Read the model definition and answer for the solid it produces. Units are mm, in the model's axes. A direction names the side the tool comes from. Give positions to 0.01 mm unless a question says otherwise; leave off trailing zeros. Order: outer loops, then holes, each group sorted by start corner. A loop starts at its lowest first (then second) coordinate and runs counter-clockwise, first axis right, second up.
```python
from build123d import *

# Parameters (mm, degrees)
F0_W      = 177.8
F0_H      = 138.684
F1_DEPTH  = 25.4
F2_W      = 177.8
F2_H      = 138.684
F2_W_2    = 161.3722443581
F2_H_2    = 112.8829941154
F3_DEPTH  = 19.05
F4_W      = 141.4277553558
F4_H      = 98.9994257689
F5_DEPTH  = 19.05
F6_R      = 25.4
F7_R      = 4.7625
F8_DEPTH  = 6.351
F9_SIZE   = 1.524
F10_R     = 1.5875
F11_DEPTH = 6.351
F12_SIZE  = 1.778


with BuildPart() as f1:
    # F0 (on Front) → F1 (new body)
    with BuildSketch(Plane.XZ):
        Rectangle(F0_W, F0_H)
    extrude(amount=F1_DEPTH)

    # F2 (on face) → F3 (cut)
    with BuildSketch(Plane(origin=(0, 0, 0), x_dir=(-1, 0, 0), z_dir=(0, 1, 0))):
        Rectangle(F2_W, F2_H)
        Rectangle(F2_W_2, F2_H_2, mode=Mode.SUBTRACT)
    extrude(amount=-F3_DEPTH, mode=Mode.SUBTRACT)

    # F4 (on face) → F5 (cut)
    with BuildSketch(Plane.XZ.offset(25.4)):
        Rectangle(F4_W, F4_H)
    extrude(amount=-F5_DEPTH, mode=Mode.SUBTRACT)

    # F6
    f6_edges = [f1.edges().sort_by_distance(p)[0] for p in [
        (88.9, -22.225, 69.342),
        (88.9, -22.225, -69.342),
        (-88.9, -22.225, -69.342),
        (-88.9, -22.225, 69.342),
        (-70.713878, -15.875, 49.499713),
        (70.713878, -15.875, 49.499713),
        (70.713878, -15.875, -49.499713),
        (-70.713878, -15.875, -49.499713),
        (80.686122, -9.525, -56.441497),
        (80.686122, -9.525, 56.441497),
        (-80.686122, -9.525, -56.441497),
        (-80.686122, -9.525, 56.441497),
    ]]
    fillet(f6_edges, radius=F6_R)

    # F7 (on face) → F8 (cut, through all)
    with BuildSketch(Plane.XZ.offset(6.35)):
        with Locations((-25.4, 23.863709036)):
            Circle(F7_R)
        with Locations((25.4, 23.863709036)):
            Circle(F7_R)
        with Locations((0, -19.9294611812)):
            Circle(F7_R)
    extrude(amount=-F8_DEPTH, mode=Mode.SUBTRACT)

    # F9
    f9_edges = [f1.edges().sort_by_distance(p)[0] for p in [
        (0, -25.4, -49.499713),
        (70.713878, -25.4, 0),
        (-88.9, -25.4, 0),
        (-81.460512, -25.4, -61.902512),
        (0, 0, -56.441497),
        (88.9, -25.4, 0),
        (81.460512, -25.4, 61.902512),
        (81.460512, -25.4, -61.902512),
        (0, -25.4, -69.342),
        (0, -25.4, 69.342),
        (-81.460512, -25.4, 61.902512),
        (-63.27439, -25.4, -42.060225),
        (63.27439, -25.4, -42.060225),
        (-70.713878, -25.4, 0),
        (-63.27439, -25.4, 42.060225),
        (63.27439, -25.4, 42.060225),
        (0, -25.4, 49.499713),
        (-80.686122, 0, 0),
        (-73.246634, 0, 49.002009),
        (-73.246634, 0, -49.002009),
        (0, 0, 56.441497),
        (73.246634, 0, 49.002009),
        (73.246634, 0, -49.002009),
        (80.686122, 0, 0),
    ]]
    chamfer(f9_edges, length=F9_SIZE)

    # F10 (on face) → F11 (cut, through all)
    with BuildSketch(Plane(origin=(0, -19.05, 0), x_dir=(-1, 0, 0), z_dir=(0, 1, 0))):
        with Locations((-79.0948867798, 54.6215597034)):
            Circle(F10_R)
        with Locations((79.6314403415, 54.6215597034)):
            Circle(F10_R)
        with Locations((79.6314403415, -54.8539970577)):
            Circle(F10_R)
        with Locations((-79.0948867798, -54.8539970577)):
            Circle(F10_R)
    extrude(amount=-F11_DEPTH, mode=Mode.SUBTRACT)

    # F12
    f12_edges = [f1.edges().sort_by_distance(p)[0] for p in [
        (-78.04394, -25.4, 54.62156),
        (80.682387, -25.4, 54.62156),
        (80.682387, -25.4, -54.853997),
        (-78.04394, -25.4, -54.853997),
    ]]
    chamfer(f12_edges, length=F12_SIZE)


solid = f1.part
```
1) Consider L1, parallel to X at y = -8.75, z = -5; L2, parallel to Z at x = -37, y = -10.5; L3, parallel to X at y = -23.75, z = 5.5. Determine where each line is inside the solid, lowest interval first.
Final values:
L1: x = -80.69 to -70.71, 70.71 to 80.69
L2: z = -56.44 to -49.5, 49.5 to 56.44
L3: x = -88.9 to -70.71, 70.71 to 88.9
2) The part is cut by section B-B on y = -15.25. Determine the outline of the cut face in (x, z).
Final values:
outline: (-80.69, -31.04) arc R25.4 ccw to (-55.29, -56.44) - (55.29, -56.44) arc R25.4 ccw to (80.69, -31.04) - (80.69, 31.04) arc R25.4 ccw to (55.29, 56.44) - (-55.29, 56.44) arc R25.4 ccw to (-80.69, 31.04) - close; hole (-70.71, -24.1) arc R25.4 ccw to (-45.31, -49.5) - (45.31, -49.5) arc R25.4 ccw to (70.71, -24.1) - (70.71, 24.1) arc R25.4 ccw to (45.31, 49.5) - (-45.31, 49.5) arc R25.4 ccw to (-70.71, 24.1) - close
3) The part is cut by section C-C on z = 12.5. Determine the outline of the cut face in (x, y), and give its area (3 significant figures).
Final values:
outline: (-88.9, -23.88) - (-87.38, -25.4) - (-72.24, -25.4) - (-70.71, -23.88) - (-70.71, -6.35) - (70.71, -6.35) - (70.71, -23.88) - (72.24, -25.4) - (87.38, -25.4) - (88.9, -23.88) - (88.9, -19.05) - (80.69, -19.05) - (80.69, -1.52) - (79.16, 0) - (-79.16, 0) - (-80.69, -1.52) - (-80.69, -19.05) - (-88.9, -19.05) - close
area: 1,500 mm2
4) The part is cut by section A-A on x = 25.4. Determine the outline of the cut face in (y, z), and give its area (3 significant figures).
Final values:
outline: (-25.4, -67.82) - (-23.88, -69.34) - (-19.05, -69.34) - (-19.05, -56.44) - (-1.52, -56.44) - (0, -54.92) - (0, 19.1) - (-6.35, 19.1) - (-6.35, -49.5) - (-23.88, -49.5) - (-25.4, -51.02) - close; (-25.4, 51.02) - (-23.88, 49.5) - (-6.35, 49.5) - (-6.35, 28.63) - (0, 28.63) - (0, 54.92) - (-1.52, 56.44) - (-19.05, 56.44) - (-19.05, 69.34) - (-23.88, 69.34) - (-25.4, 67.82) - close
area: 1,080 mm2
5) Given pin 1 (3.5 mm diameter, centred on x = -79.63, z = 54.62, fed in from -Y); pin 2 (10 mm diameter, centred on y = -18.5, z = 40.5, fed in from -X); pin 3 (12.5 mm diameter, centred on x = 0, z = -19.93, fed in from -Y); pin 4 (14 mm diameter, centred on y = -9, z = -8, fed in from -X), each flat-ended and moving along its own axis, determine where each tip first touches the part or whether it passes through.
Final values:
pin 1: stops at y = -23.79
pin 2: stops at x = -88.9
pin 3: stops at y = -6.35
pin 4: stops at x = -80.69
6) A tool of negligible diameter and unlimited length cuts with its end or side. For faces 5 (the face through (70.714, -15, 0)), 6 (the face through (1, -10, -56.441)), 7 (the face through (73.048, -10.41, 49.198)), from which of +Z, -Z, +X, -X, +Y, -Y can it reach the whole face along a straight path? Write none if from no direction.
Final values:
face 5: -Y
face 6: -Z, +X, -X, +Y
face 7: +Z, +X, +Y
7) The part is cut by section D-D on x = -38.5. Determine the outline of the cut face in (y, z).
Final values:
outline: (-25.4, -67.82) - (-23.88, -69.34) - (-19.05, -69.34) - (-19.05, -56.44) - (-1.52, -56.44) - (0, -54.92) - (0, 54.92) - (-1.52, 56.44) - (-19.05, 56.44) - (-19.05, 69.34) - (-23.88, 69.34) - (-25.4, 67.82) - (-25.4, 51.02) - (-23.88, 49.5) - (-6.35, 49.5) - (-6.35, -49.5) - (-23.88, -49.5) - (-25.4, -51.02) - close
8) For a pull along X with two mould halves and no side action, classify faces 1 (the face through (88.9, -21, -1)), 2 (the face through (-81.66, -21.5, -61.7)), 3 (the face through (-1, -6.35, 1)), 4 (the face through (-1, -15, -49.5)) as released by +X, released by -X, zero draft, split by the parting line, or undercut.
Final values:
face 1: released by +X
face 2: released by -X
face 3: undercut
face 4: undercut
